Study the drawing (mm; zero at the part's minimum x, y, z) and answer. Coordinates: 2 decimals unless noted, no trailing zeros. Order: outer loops, then holes, each group sorted by start corner. A loop starts at its lowest first (then second) coordinate and runs counter-clockwise, first axis right, second up.
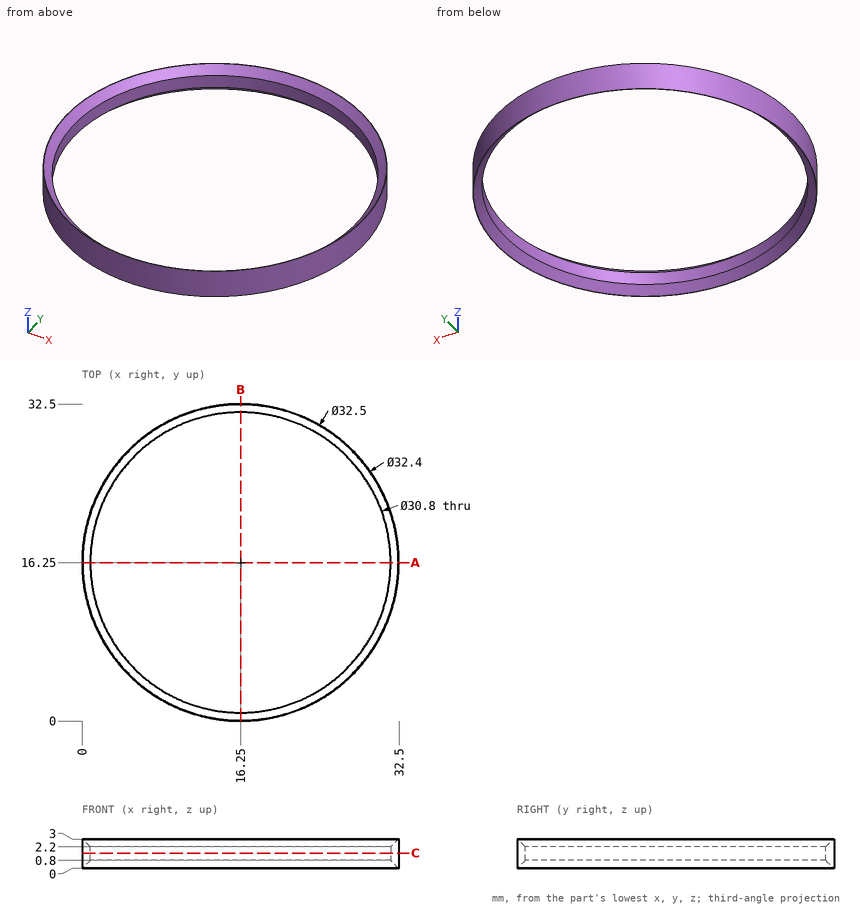
1) A flat-ended cylindrical pin translates along its axis: pin 1 Ø1.5 at (x, z) = (9.5, 1.5) entering from +Y. Find the tip coordinate at first contact, or state that the pin passes through.
A:
pin 1: stops at y = 31.35
2) Straight lines are drawn through the part: line 1 (Y direction, x = 16.25, z = 1.9); line 2 (Y direction, x = 21.5, z = 0.3). For each, find the intervals that lie inside material, in ascending order.
A:
line 1: y = 0 to 0.85, 31.65 to 32.5
line 2: y = 0.87 to 1.24, 31.26 to 31.63
3) A cutting plane is placed at A-A, the plane y = 16.25. Determine the outline of the cut face in (x, z).
A:
outline: (0, 0) - (0.05, 0) - (0.85, 0.8) - (0.85, 2.2) - (0.05, 3) - (0, 3) - close; (31.65, 0.8) - (32.45, 0) - (32.5, 0) - (32.5, 3) - (32.45, 3) - (31.65, 2.2) - close
4) A cutting plane is placed at C-C, the plane z = 1.55. Determine the outline of the cut face in (x, y).
A:
outline: circle Ø32.5 at (16.25, 16.25); hole circle Ø30.8 at (16.25, 16.25)
